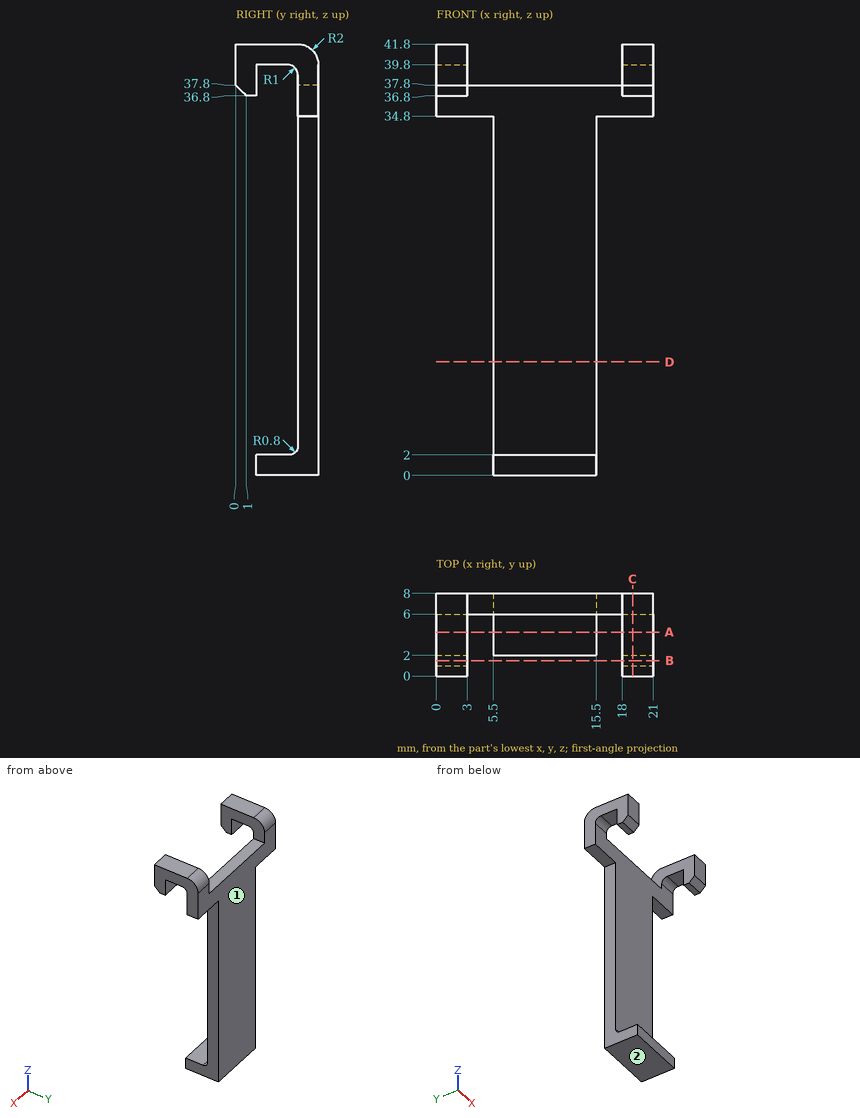
Input: dimensioned drawing with shaded views. Units: mm. Origin: part minimum x, y, z. Round coordinates to 2 decimals unless told otherwise and drop trailing zeros. Loops run counter-clockwise (first coordinate to the right, second up) from the corner with the lowest first, then second, coordinate; pieces in that order, holes last.
1) Section query B-B on y = 1.5. Return the cut outline in (x, z).
Ans:
outline: (0, 36.8) - (3, 36.8) - (3, 41.8) - (0, 41.8) - close; (18, 36.8) - (21, 36.8) - (21, 41.8) - (18, 41.8) - close
2) Pull-direction query (Y, two-part tool) for the marked faces 1 and 2; classes: released by +Y, released by -Y, zero draft, split by the parting line, or undercut.
Ans:
face 1: released by +Y
face 2: zero draft
3) Material intervals for line 1 (Y direction, x = 13, z = 26); line 2 (Z direction, x = 8, y = 6.5); line 3 (Z direction, x = 20.25, y = 4.5), sorted ascending.
Ans:
line 1: y = 6 to 8
line 2: z = 0 to 37.8
line 3: z = 39.8 to 41.8
4) Section query C-C on x = 19. Return the cut outline in (y, z), plus the area to 3 significant figures.
Ans:
outline: (0, 37.8) - (1, 36.8) - (2, 36.8) - (2, 39.8) - (5, 39.8) arc R1 cw to (6, 38.8) - (6, 34.8) - (8, 34.8) - (8, 39.8) arc R2 ccw to (6, 41.8) - (0, 41.8) - close
area: 30.9 mm2
5) Section query D-D on z = 11. Return the cut outline in (x, y), plus the area to 3 significant figures.
Ans:
outline: (5.5, 6) - (15.5, 6) - (15.5, 8) - (5.5, 8) - close
area: 20.0 mm2
6) Pin query (flat end, axial travel): pin 1 (3.5 mm diameter, centred on x = 19.5, y = 4, fed in from -Z); pin 2 (0.6 mm diameter, centred on x = 17.5, y = 7.5, fed in from -Z); pin 3 (0.5 mm diameter, centred on x = 19, y = 1.5, fed in from -Z). Return the tip coordinate at first contact, or that it passes through.
Ans:
pin 1: stops at z = 39.46
pin 2: stops at z = 34.8
pin 3: stops at z = 36.8
7) Section query A-A on y = 4.25. Return the cut outline in (x, z).
Ans:
outline: (0, 39.8) - (3, 39.8) - (3, 41.8) - (0, 41.8) - close; (5.5, 0) - (15.5, 0) - (15.5, 2) - (5.5, 2) - close; (18, 39.8) - (21, 39.8) - (21, 41.8) - (18, 41.8) - close
